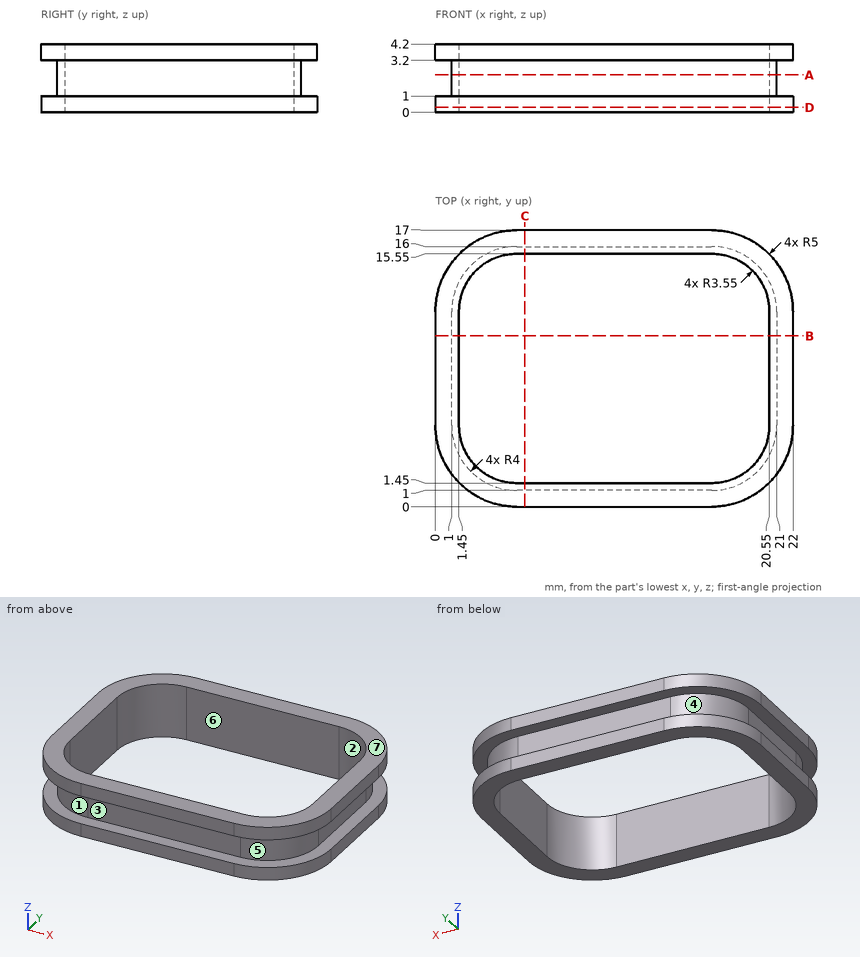
Geometry check sheet. Reference: drawing and pictorial views, mm from the part's lowest x, y, z. A direction names the side the tool comes from. Give positions to 0.01 mm unless a question says otherwise; leave off trailing zeros. Write each loop counter-clockwise with the first axis right and the second up, starting at its lowest first coordinate (ties: lowest second). Pieces come first, ordered by that corner, then holes. Notation, with made-up numbers: (69, 70.25) -> (105, 70.25) arc R18 ccw to (105, 98.25) -> close; hole circle Ø8 at (69, 56.25). An arc over 180 degrees is marked (long way). One line per item, written item: value. Start each with the question number.
Item 1: Section check D-D on z = 0.3. Record the cut outline in (x, y), then the cut area to 3 significant figures.
Item 2: Section check B-B on y = 10.5. Record the cut outline in (x, z).
Item 3: Gauge pin test, flat ends, axial feed: pin 1 (1 mm diameter, centred on x = 10, y = 3, fed in from +Z); pin 2 (8.5 mm diameter, centred on x = 13.5, y = 12.5, fed in from -Z); pin 3 (0.7 mm diameter, centred on x = 9, z = 2.5, fed in from -Y); pin 4 (0.7 mm diameter, centred on y = 7, z = 2, fed in from +X). Record the tip position at first contact, or that the pin passes through.
Item 4: Draft check along X on the marked faces 5, 6 and 7. Enter one of: +X half, -X half, draft (parallel to the pull), parting line (faces both ways), or undercut.
Item 5: Material ranges on probe 1 along X at (y, z) = (9.5, 3.9); probe 2 along Y at (x, z) = (6, 1.95); probe 3 along X at (y, z) = (9, 1.7), recorded low to high. Write a range as from..to.
Item 6: Tool access check on the marked faces 1, 2, 3 and 4. Record the directions out of +Z, -Z, +X, -X, +Y, -Y that give a thin tool (end or side, any length) a straight path to the whole face; none if there is none.
Item 7: Section check C-C on x = 5.5. Record the cut outline in (y, z).
Item 8: Section check A-A on z = 2.3. Record the cut outline in (x, y), then the cut area to 3 significant figures.
Results list:
1. outline: (0, 5) arc R5 ccw to (5, 0) -> (17, 0) arc R5 ccw to (22, 5) -> (22, 12) arc R5 ccw to (17, 17) -> (5, 17) arc R5 ccw to (0, 12) -> close; hole (1.45, 5) arc R3.55 ccw to (5, 1.45) -> (17, 1.45) arc R3.55 ccw to (20.55, 5) -> (20.55, 12) arc R3.55 ccw to (17, 15.55) -> (5, 15.55) arc R3.55 ccw to (1.45, 12) -> close
1. area: 94.0 mm²
2. outline: (0, 0) -> (1.45, 0) -> (1.45, 4.2) -> (0, 4.2) -> (0, 3.2) -> (1, 3.2) -> (1, 1) -> (0, 1) -> close; (20.55, 0) -> (22, 0) -> (22, 1) -> (21, 1) -> (21, 3.2) -> (22, 3.2) -> (22, 4.2) -> (20.55, 4.2) -> close
3. pin 1: through
3. pin 2: z = 0
3. pin 3: y = 1
3. pin 4: x = 21
4. face 5: +X half
4. face 6: undercut
4. face 7: draft
5. probe 1: 0..1.45, 20.55..22
5. probe 2: 1..1.45, 15.55..16
5. probe 3: 1..1.45, 20.55..21
6. face 1: -X, -Y
6. face 2: +Z, -Z
6. face 3: +X, -X, -Y
6. face 4: -X, +Y
7. outline: (0, 0) -> (1.45, 0) -> (1.45, 4.2) -> (0, 4.2) -> (0, 3.2) -> (1, 3.2) -> (1, 1) -> (0, 1) -> close; (15.55, 0) -> (17, 0) -> (17, 1) -> (16, 1) -> (16, 3.2) -> (17, 3.2) -> (17, 4.2) -> (15.55, 4.2) -> close
8. outline: (1, 5) arc R4 ccw to (5, 1) -> (17, 1) arc R4 ccw to (21, 5) -> (21, 12) arc R4 ccw to (17, 16) -> (5, 16) arc R4 ccw to (1, 12) -> close; hole (1.45, 5) arc R3.55 ccw to (5, 1.45) -> (17, 1.45) arc R3.55 ccw to (20.55, 5) -> (20.55, 12) arc R3.55 ccw to (17, 15.55) -> (5, 15.55) arc R3.55 ccw to (1.45, 12) -> close
8. area: 27.8 mm²
